Geometry check sheet. Reference: the model listing, model coordinates, mm. A direction names the side the tool comes from. Round coordinates to 2 decimals unless told otherwise and drop trailing zeros. Write each loop counter-clockwise with the first axis right and the second up, starting at its lowest first coordinate (ties: lowest second). Pieces come first, ordered by that corner, then holes. Notation, with made-up numbers: (53.25, -23.5) - (76.25, -23.5) arc R21 ccw to (76.25, -7.5) - close; hole circle Ø6 at (44.25, 10). An arc over 180 degrees is marked (long way). Return JSON: item names as keys, results as strings. Group by question number.
from build123d import *

# Parameters (mm, degrees)
SKETCH1_W             = 60
SKETCH1_H             = 15
BASE_FLANGE1_DEPTH    = 0.7
EDGE_FLANGE1_DEPTH    = 55
CUT_EXTRUDE1_DEPTH    = 46.250862749
BREAK_CORNER1_START   = -0.7
BREAK_CORNER1_DEPTH   = 0.7
BREAK_CORNER1_START_2 = 8.2366
BREAK_CORNER1_2_DEPTH = 0.7


# Read off the part's stored shape, not the designer's step: Break-Corner1
# Sheet-metal steps are written as plain solids
with BuildPart() as part:
    # Sketch1 → Base-Flange1 (new body)
    with BuildSketch(Plane(origin=(0, 0, 0), x_dir=(1, 0, 0), z_dir=(0, 1, 0))):
        Rectangle(SKETCH1_W, SKETCH1_H)
    extrude(amount=-BASE_FLANGE1_DEPTH)

    # Edge-Flange1 section (across the edge) → Edge-Flange1 (add)
    with BuildSketch(Plane(origin=(-27.5, 0, 8.2366), x_dir=(0, 0, -1), z_dir=(1, 0, 0))):
        with BuildLine():
            Line((-0.7, 0.7366), (-0.7, 30))
            Line((-0.7, 30), (0, 30))
            Line((0, 30), (0, 0.7366))
            ThreePointArc((0, 0.7366), (0.215745145, 0.215745145), (0.7366, 0))
            Line((0.7366, 0), (0.7366, -0.7))
            ThreePointArc((0.7366, -0.7), (-0.279229602, -0.279229602), (-0.7, 0.7366))
        make_face()
    extrude(amount=EDGE_FLANGE1_DEPTH)

    # Sketch7 → Cut-Extrude1 (cut, through all)
    with BuildSketch(Plane(origin=(0, 0, 8.2366), x_dir=(-1, 0, 0), z_dir=(0, 0, -1))):
        with BuildLine():
            Line((-15.8, 25), (-15.8, 5))
            ThreePointArc((-15.8, 5), (-17.5, 3.3), (-19.2, 5))
            Line((-19.2, 5), (-19.2, 25))
            ThreePointArc((-19.2, 25), (-17.5, 26.7), (-15.8, 25))
        make_face()
        with BuildLine():
            Line((19.2, 25), (19.2, 5))
            ThreePointArc((19.2, 5), (17.5, 3.3), (15.8, 5))
            Line((15.8, 5), (15.8, 25))
            ThreePointArc((15.8, 25), (17.5, 26.7), (19.2, 25))
        make_face()
    extrude(amount=-CUT_EXTRUDE1_DEPTH, mode=Mode.SUBTRACT)

    # Break-Corner1 outline → Break-Corner1 (cut)
    with BuildSketch(Plane(origin=(0, 0, 0), x_dir=(1, 0, 0), z_dir=(0, 1, 0)).offset(BREAK_CORNER1_START)):
        with BuildLine():
            ThreePointArc((-27.501, -7.5), (-29.268059846, -6.768059846), (-30, -5.001))
            Line((-30, -5.001), (-30, -7.5))
            Line((-30, -7.5), (-27.501, -7.5))
        make_face()
        with BuildLine():
            ThreePointArc((-30, 5.001), (-29.268059846, 6.768059846), (-27.501, 7.5))
            Line((-27.501, 7.5), (-30, 7.5))
            Line((-30, 7.5), (-30, 5.001))
        make_face()
        with BuildLine():
            ThreePointArc((27.501, 7.5), (29.268059846, 6.768059846), (30, 5.001))
            Line((30, 5.001), (30, 7.5))
            Line((30, 7.5), (27.501, 7.5))
        make_face()
        with BuildLine():
            ThreePointArc((30, -5.001), (29.268059846, -6.768059846), (27.501, -7.5))
            Line((27.501, -7.5), (30, -7.5))
            Line((30, -7.5), (30, -5.001))
        make_face()
    extrude(amount=BREAK_CORNER1_DEPTH, mode=Mode.SUBTRACT)

    # Break-Corner1 2 outline → Break-Corner1 2 (cut)
    with BuildSketch(Plane.XY.offset(BREAK_CORNER1_START_2)):
        with BuildLine():
            Line((-27.5, 30), (-27.5, 27.501))
            ThreePointArc((-27.5, 27.501), (-26.768059846, 29.268059846), (-25.001, 30))
            Line((-25.001, 30), (-27.5, 30))
        make_face()
        with BuildLine():
            Line((27.5, 30), (25.001, 30))
            ThreePointArc((25.001, 30), (26.768059846, 29.268059846), (27.5, 27.501))
            Line((27.5, 27.501), (27.5, 30))
        make_face()
    extrude(amount=BREAK_CORNER1_2_DEPTH, mode=Mode.SUBTRACT)


solid = part.part
1. Section check C-C (z = -0.75). Enter the section's corners in (x, y), and give its area (3 significant figures).
2. Depth check by flat-ended pin: pin 1 Ø14.5 at (x, y) = (-1.5, 17) entering from -Z; pin 2 Ø0.6 at (y, z) = (15.5, 8.5) entering from +X; pin 3 Ø4 at (x, z) = (-1, 3.5) entering from +Y. Enter the tip coordinate at first touch or a pass-through.
3. Tool access check on faces 1 (the face through (17.5, 3.3, 8.6)), 2 (the face through (29.249, -0.355, -6.787)), 3 (the face through (0, 16, 8.237)). Record the directions out of +Z, -Z, +X, -X, +Y, -Y that give a thin tool (end or side, any length) a straight path to the whole face; none if there is none.
4. Section check B-B (y = 7). Enter the section's corners in (x, z), and give its area (3 significant figures).
5. Section check A-A (x = -17.5). Enter the section's corners in (y, z), and give its area (3 significant figures).
6. Mould release check, pull along Y, two halves, no side actions. Record for faces 4 (the face through (29.287, -0.355, 6.749)), 5 (the face through (-17.5, 26.7, 8.6)), 6 (the face through (26.749, 29.287, 8.582)), 7 (the face through (17.5, 26.7, 8.6)): pulls with the +Y half, pulls with the -Y half, needs draft (parallel to the pull), parting line crosses it, or undercut.
7. Material ranges on line 1 along Z through (x, y) = (23.5, 25); line 2 along Y through (x, z) = (-19.5, -5.25), recorded low to high.
Result sheet:
{
 "1": {"outline": "(-30, -0.7) - (30, -0.7) - (30, 0) - (-30, 0) - close", "area": "42.0 mm²"},
 "2": {"pin 1": "stops at z = 8.24", "pin 2": "stops at x = 27.5", "pin 3": "stops at y = 0"},
 "3": {"face 1": "+Z, -Z", "face 2": "-Z, +X, +Y, -Y", "face 3": "-Z, +X, -X, +Y"},
 "4": {"outline": "(-27.5, 8.24) - (-19.2, 8.24) - (-19.2, 8.94) - (-27.5, 8.94) - close; (-15.8, 8.24) - (15.8, 8.24) - (15.8, 8.94) - (-15.8, 8.94) - close; (19.2, 8.24) - (27.5, 8.24) - (27.5, 8.94) - (19.2, 8.94) - close", "area": "33.7 mm²"},
 "5": {"outline": "(-0.7, -7.5) - (0, -7.5) - (0, 7.5) arc R0.74 cw to (0.74, 8.24) - (3.3, 8.24) - (3.3, 8.94) - (0.74, 8.94) arc R1.44 ccw to (-0.7, 7.5) - close; (26.7, 8.24) - (30, 8.24) - (30, 8.94) - (26.7, 8.94) - close", "area": "15.8 mm²"},
 "6": {"face 4": "needs draft", "face 5": "undercut", "face 6": "pulls with the +Y half", "face 7": "undercut"},
 "7": {"line 1": "z = 8.24 to 8.94", "line 2": "y = -0.7 to 0"}
}
